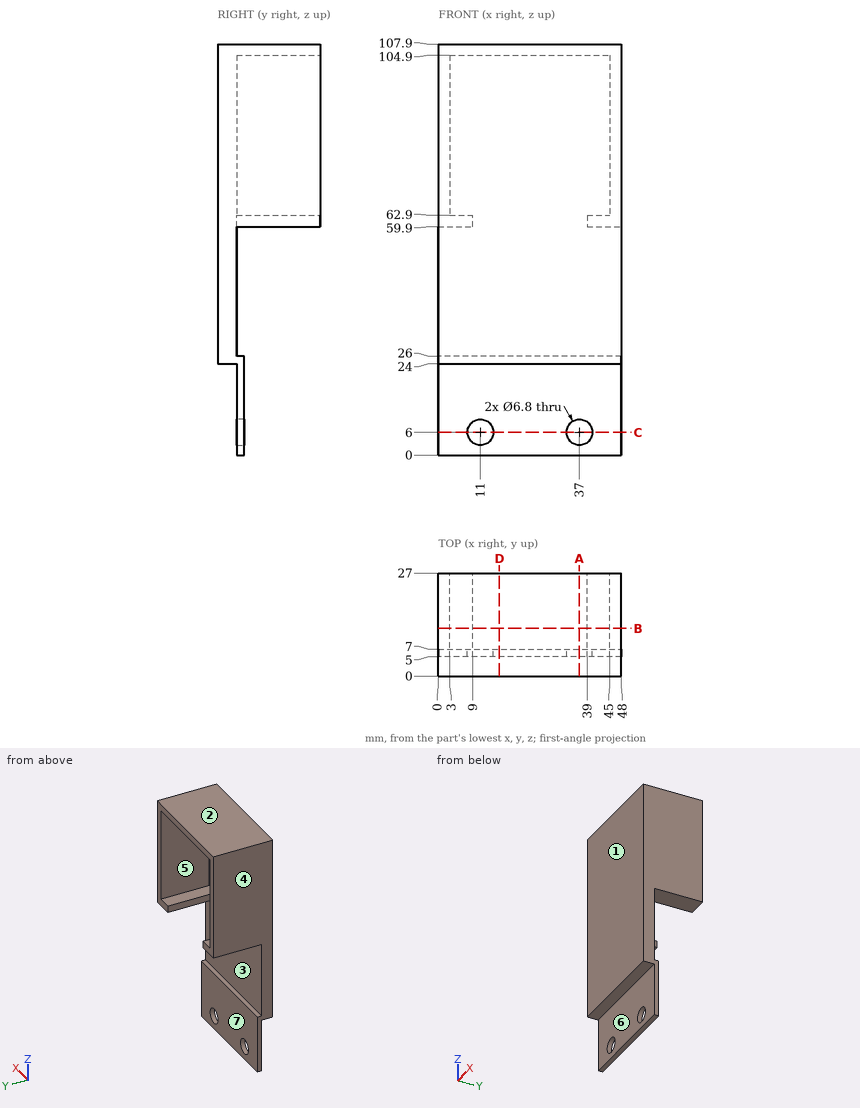
Input: dimensioned drawing with shaded views. Units: mm. Origin: part minimum x, y, z. A direction names the side the tool comes from. Give positions to 0.01 mm unless a question says otherwise; leave off trailing zeros. Order: outer loops, then holes, each group sorted by start corner. A loop starts at its lowest first (then second) coordinate and runs counter-clockwise, first axis right, second up.
(1) Contact query for flat-ended pins moving along their axis: P1, Ø11, axis at x = 13.5, y = 20, coming from the -Z side; P2, Ø4, axis at x = 19, y = 3.5, coming from the -Z side; P3, Ø19, axis at x = 31, z = 7, coming from the -Y side; P4, Ø14.5, axis at x = 20.5, z = 70, coming from the +Y side. Output: stop coordinate, or through.
(2) Pull-direction query (Z, two-part tool) for the marked faces 1, 2 and 3; classes: +Z half, -Z half, draft (parallel to the pull), parting line (faces both ways), or undercut.
(3) Section query A-A (x = 37). Return the cut outline in (y, z), plus the area to 3 significant figures.
(4) Section query B-B (y = 12.5). Return the cut outline in (x, z), plus the area to 3 significant figures.
(5) Section query C-C (z = 6). Return the cut outline in (x, y), plus the area to 3 significant figures.
(6) Material intervals for line 1 along X through (y, z) = (5.7, 6); line 2 along X through (y, z) = (24.75, 73); line 3 along Z through (x, y) = (4, 17.5), sorted ascending.
(7) Access query for the marked faces 4, 5, 6 and 7. Directions: +Z, -Z, +X, -X, +Y, -Y. A direction counts if a zero-diameter tool reaches every point of the face in a straight line with its end or side. Return the directions, or none.
(8) Section query D-D (x = 16). Return the cut outline in (y, z).
Outcome:
1. P1: stops at z = 59.9
1. P2: stops at z = 0
1. P3: stops at y = 5
1. P4: stops at y = 5
2. face 1: draft
2. face 2: +Z half
2. face 3: undercut
3. outline: (0, 24) - (5, 24) - (5, 9.4) - (7, 9.4) - (7, 26) - (5, 26) - (5, 104.9) - (27, 104.9) - (27, 107.9) - (0, 107.9) - close; (5, 0) - (7, 0) - (7, 2.6) - (5, 2.6) - close
3. area: 524 mm2
4. outline: (0, 59.9) - (9, 59.9) - (9, 62.9) - (3, 62.9) - (3, 104.9) - (45, 104.9) - (45, 62.9) - (39, 62.9) - (39, 59.9) - (48, 59.9) - (48, 107.9) - (0, 107.9) - close
4. area: 450 mm2
5. outline: (0, 5) - (7.6, 5) - (7.6, 7) - (0, 7) - close; (14.4, 5) - (33.6, 5) - (33.6, 7) - (14.4, 7) - close; (40.4, 5) - (48, 5) - (48, 7) - (40.4, 7) - close
5. area: 68.8 mm2
6. line 1: x = 0 to 7.6, 14.4 to 33.6, 40.4 to 48
6. line 2: x = 0 to 3, 45 to 48
6. line 3: z = 59.9 to 62.9, 104.9 to 107.9
7. face 4: +Z, -Z, -X, +Y, -Y
7. face 5: +Y
7. face 6: -Z, +X, -X, -Y
7. face 7: -Z, +X, -X, +Y
8. outline: (0, 24) - (5, 24) - (5, 0) - (7, 0) - (7, 26) - (5, 26) - (5, 104.9) - (27, 104.9) - (27, 107.9) - (0, 107.9) - close
